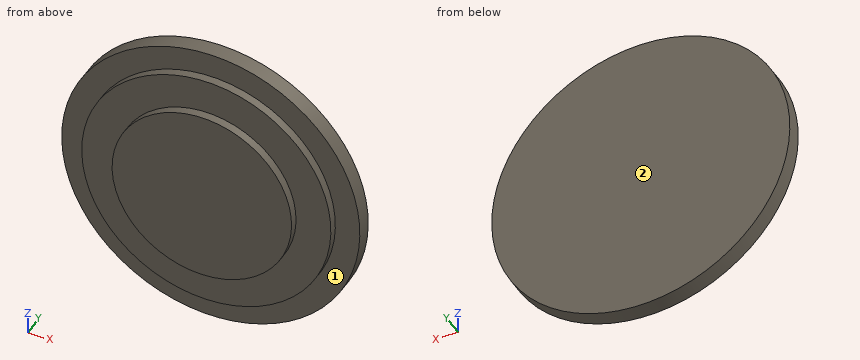
from build123d import *

# Parameters (mm, degrees)
SKETCH_1_W      = 137
SKETCH_1_H      = 15
SKETCH_2_R      = 114.5
EXTRUDE_1_DEPTH = 8
SKETCH_3_R      = 82.5
EXTRUDE_2_DEPTH = 8


with BuildPart() as part:
    # 草圖1 → 旋轉1 (revolve)
    with BuildSketch(Plane(origin=(0, 0, 0), x_dir=(-1, 0, 0), z_dir=(0, 0, -1)), mode=Mode.PRIVATE) as revolve_1_sk:
        with Locations((-68.5, 35.5)):
            Rectangle(SKETCH_1_W, SKETCH_1_H)
    revolve(revolve_1_sk.sketch.rotate(Axis((0, 28, 0), (0, 1, 0)), 270), axis=Axis((0, 28, 0), (0, 1, 0)))

    # 草圖2 → 填料-伸長1 (add)
    with BuildSketch(Plane.XZ.offset(-28)):
        with Locations(Location((0, 0, 0), (0, 0, 270))):
            Circle(SKETCH_2_R)
    extrude(amount=EXTRUDE_1_DEPTH)

    # 草圖3 → 填料-伸長2 (add)
    with BuildSketch(Plane.XZ.offset(-20)):
        with Locations(Location((0, 0, 0), (0, 0, 270))):
            Circle(SKETCH_3_R)
    extrude(amount=EXTRUDE_2_DEPTH)


solid = part.part
Input: part model. Units: mm. Frame: model coordinates. Face numbers are marked on the shaded views. A direction names the side the tool comes from. Give positions to 0.01 mm unless a question says otherwise; leave off trailing zeros. Order: outer loops, then holes, each group sorted by start corner. A loop starts at its lowest first (then second) coordinate and runs counter-clockwise, first axis right, second up. Notation, with made-up numbers: (-39.75, 25) - (-17.75, 25) arc R23 ccw to (-17.75, 60) - close; hole circle Ø8 at (18.25, 83). An arc over 180 degrees is marked (long way). Answer as a JSON object with one key per item and string values. Group by question number.
Q1. Cut plane B-B, the plane z = 0. Output: boundary loops of the cut face in (x, y).
Q2. Cut plane A-A, the plane x = 0. Output: boundary loops of the cut face in (y, z), then the cut area to 3 significant figures.
Q3. Line query: probe 1 along Y at (x, z) = (125, 36); probe 2 along Y at (x, z) = (12, 86); probe 3 along Z at (x, y) = (-1.5, 14). Output: solid intervals per line, ascending.
Q4. Set-up query: the marked faces 1 and 2. Return all of +Z, -Z, +X, -X, +Y, -Y with unobstructed straight access to the full face (end or side cutting, diameter ignored); none if empty.
Q5. First-contact query: pin 1 Ø1 at (x, y) = (86, 22) entering from +Z; pin 2 Ø12 at (x, y) = (-69.5, 28.5) entering from +Z (3 decimals); pin 3 Ø8 at (y, z) = (33, -32.5) entering from -X. Flat tips, straight axial feed; report the tip coordinate or a pass-through.
Q6. Cut plane C-C, the plane y = 35.5. Output: boundary loops of the cut face in (x, z), then the cut area to 3 significant figures.
Q7. Cut plane D-D, the plane z = 110. Output: boundary loops of the cut face in (x, y).
Results:
{
 "1": {"outline": "(-137, 28) - (-114.5, 28) - (-114.5, 20) - (-82.5, 20) - (-82.5, 12) - (82.5, 12) - (82.5, 20) - (114.5, 20) - (114.5, 28) - (137, 28) - (137, 43) - (-137, 43) - close"},
 "2": {"outline": "(12, -82.5) - (20, -82.5) - (20, -114.5) - (28, -114.5) - (28, -137) - (43, -137) - (43, 137) - (28, 137) - (28, 114.5) - (20, 114.5) - (20, 82.5) - (12, 82.5) - close", "area": "7,260 mm^2"},
 "3": {"probe 1": "28 to 43", "probe 2": "20 to 43", "probe 3": "-82.49 to 82.49"},
 "4": {"face 1": "-Y", "face 2": "+Z, -Z, +X, -X, +Y"},
 "5": {"pin 1": "z = 76.16", "pin 2": "z = 121.395", "pin 3": "x = -134"},
 "6": {"outline": "circle Ø274 at (0, 0)", "area": "59,000 mm^2"},
 "7": {"outline": "(-81.66, 28) - (-31.78, 28) - (-31.78, 20) - (31.78, 20) - (31.78, 28) - (81.66, 28) - (81.66, 43) - (-81.66, 43) - close"}
}
